from build123d import *

# Parameters (mm, degrees)
SKETCH_1_R          = 2.7
EXTRUDE_1_DEPTH     = 1.7
CUT_EXTRUDE_1_DEPTH = 0.5
SKETCH_3_R          = 1.5
EXTRUDE_2_DEPTH     = 6


with BuildPart() as part:
    # 草图1 → 凸台-拉伸1 (new body)
    with BuildSketch(Plane(origin=(0, 0, 0), x_dir=(1, 0, 0), z_dir=(0, 1, 0))):
        with Locations(Location((0, 0, 0), (0, 0, 270))):
            Circle(SKETCH_1_R)
    extrude(amount=EXTRUDE_1_DEPTH)

    # 草图2 → 切除-拉伸1 (cut)
    with BuildSketch(Plane(origin=(0, 1.7, 0), x_dir=(1, 0, 0), z_dir=(0, 1, 0))):
        Polygon((0, 1.5), (0.5, 1.5), (0.5, 0.5), (1.5, 0.5), (1.5, 0), (1.5, -0.5), (0.5, -0.5), (0.5, -1.5), (0, -1.5), (-0.5, -1.5), (-0.5, -0.5), (-1.5, -0.5), (-1.5, 0), (-1.5, 0.5), (-0.5, 0.5), (-0.5, 1.5), align=None)
    extrude(amount=-CUT_EXTRUDE_1_DEPTH, mode=Mode.SUBTRACT)

    # 草图3 → 凸台-拉伸2 (add)
    with BuildSketch(Plane.XZ):
        with Locations(Location((0, 0, 0), (0, 0, 270))):
            Circle(SKETCH_3_R)
    extrude(amount=EXTRUDE_2_DEPTH)


solid = part.part
The model under review builds one solid part; all positions refer to its coordinate system, in mm. A direction names the side the tool comes from. Give positions to 0.01 mm unless a question says otherwise; leave off trailing zeros. Order: outer loops, then holes, each group sorted by start corner. A loop starts at its lowest first (then second) coordinate and runs counter-clockwise, first axis right, second up. Notation, with made-up numbers: M 67.5,76 L 123.5,76 A21 cw 123.5,113 Z; hole C -28,85.5 d11. An arc over 180 degrees is marked long. Answer in a Markdown table with one row per item. Add a question column.
1. Add section B-B on x = 0. State the section outline as (y, z) points, plus the area to 3 significant figures.
2. Machinability: for faces 1 (the flat face through (-1, 1.7, 1)), 2 (the flat face through (-1.2, 0, 1.2)), which of the approach directions +Z, -Z, +X, -X, +Y, -Y give a long, thin tool a straight path to every point of the face, cutting with its end or side? Answer none if there is none.
3. For pin 1 Ø1.5 at (x, y) = (1, -2) entering from -Z; pin 2 Ø0.6 at (y, z) = (1.5, -1) entering from -X; pin 3 Ø1.5 at (x, z) = (2, 2) entering from -Y, all flat-tipped, find the tip position at first contact; note any pin that passes through.
4. Add section A-A on z = 0. State the section outline as (x, y) points, plus the area to 3 significant figures.
5. Add section D-D on z = 1.7. State the section outline as (x, y) points.
6. To check wall thickness, follow line 1 along X through (y, z) = (1.5, -0.1); line 2 along Y through (x, z) = (0.3, 0.25); line 3 along Y through (x, z) = (1.45, 1.2). State the ranges of each line that lie inside material, in increasing order.
7. Add section C-C on y = -1.5. State the section outline as (x, z) points.
8. Mouldability with a two-part tool opening along Z and no side actions: class faces 3 (the flat face through (0, 1.2, 0)), 4 (the cylindrical face through (0.811, 0.838, 2.575)), 5 (the flat face through (0, -6, 0)) as released by +Z, released by -Z, zero draft, split by the parting line, or undercut.
The answers:
| question | item | result |
|---|---|---|
| 1 | outline | M -6,-1.5 L 0,-1.5 L 0,-2.7 L 1.7,-2.7 L 1.7,-1.5 L 1.2,-1.5 L 1.2,1.5 L 1.7,1.5 L 1.7,2.7 L 0,2.7 L 0,1.5 L -6,1.5 Z |
| 1 | area | 25.7 mm2 |
| 2 | face 1 | +Z, -Z, +X, -X, +Y |
| 2 | face 2 | -Y |
| 3 | pin 1 | z = -1.48 |
| 3 | pin 2 | x = -2.61 |
| 3 | pin 3 | y = 0 |
| 4 | outline | M -2.7,0 L -1.5,0 L -1.5,-6 L 1.5,-6 L 1.5,0 L 2.7,0 L 2.7,1.7 L 1.5,1.7 L 1.5,1.2 L -1.5,1.2 L -1.5,1.7 L -2.7,1.7 Z |
| 4 | area | 25.7 mm2 |
| 5 | outline | M -2.1,0 L 2.1,0 L 2.1,1.7 L -2.1,1.7 Z |
| 6 | line 1 | -2.7 to -1.5, 1.5 to 2.7 |
| 6 | line 2 | -6 to 1.2 |
| 6 | line 3 | 0 to 1.7 |
| 7 | outline | C 0,0 d3 |
| 8 | face 3 | undercut |
| 8 | face 4 | split by the parting line |
| 8 | face 5 | zero draft |
